CAD build for the part. Positions are in the model's coordinates, mm. A direction names the side the tool comes from. Give positions to 0.01 mm unless a question says otherwise; leave off trailing zeros. Loops run counter-clockwise (first coordinate to the right, second up) from the corner with the lowest first, then second, coordinate; pieces in that order, holes last.
```python
from build123d import *

# Parameters (mm, degrees)
F1_DEPTH = 2
F2_DEPTH = 14
F3_DEPTH = 4
F4_DEPTH = 14
F5_R     = 5


with BuildPart() as f1:
    # F0 (on Front) → F1 (new body)
    with BuildSketch(Plane.XZ):
        Polygon((26.906193, 0), (-25.108696, 0), (-25.108696, -13), (26.906193, -7.798511), align=None)
        Polygon((-25.108696, 10), (-25.108696, 0), (26.906193, 0), (26.906193, 4.798511), align=None)
    extrude(amount=F1_DEPTH)

    # F0 (on Front) → F2 (join)
    with BuildSketch(Plane.XZ):
        Polygon((26.906193, 4.798511), (26.906193, 0), (29.891304, 0), (29.891304, 15), (26.906193, 15), (26.906193, 7.798511), align=None)
    extrude(amount=F2_DEPTH)

    # F0 (on Front) → F3 (join)
    with BuildSketch(Plane.XZ):
        Polygon((-25.108696, 13), (-25.108696, 10), (26.906193, 4.798511), (26.906193, 7.798511), align=None)
    extrude(amount=F3_DEPTH)

    # F0 (on Front) → F4 (join)
    with BuildSketch(Plane.XZ):
        Polygon((29.891304, 0), (26.906193, 0), (26.906193, -7.798511), (26.906193, -15), (29.891304, -15), align=None)
    extrude(amount=F4_DEPTH)

    # F5
    f5_edges = [f1.edges().sort_by_distance(p)[0] for p in [
        (28.398748, -14, -15),
        (28.398748, -14, 15),
    ]]
    fillet(f5_edges, radius=F5_R)


solid = f1.part
```
1. Saw through at D-D, the plane y = -7.25. List the corners of the cut face in (x, z).
Responses:
outline: (26.91, -15) - (29.89, -15) - (29.89, 15) - (26.91, 15) - close
2. Saw through at C-C, the plane x = 18.5. List the corners of the cut face in (y, z), and give its area (3 significant figures).
Responses:
outline: (-4, 5.64) - (-2, 5.64) - (-2, -8.64) - (0, -8.64) - (0, 8.64) - (-4, 8.64) - close
area: 40.6 mm2
3. Drop flat-ended pins along their axis: pin 1 (10 mm diameter, centred on x = -6.5, z = -7, fed in from -Y); pin 2 (1 mm diameter, centred on y = -3, z = -12, fed in from -X); pin 3 (6.5 mm diameter, centred on x = -4.5, z = 8.5, fed in from -Y). Give the stop position or say it passes through.
Responses:
pin 1: stops at y = -2
pin 2: stops at x = 26.91
pin 3: stops at y = -4
4. Probe line 1 along Y through (x, z) = (8.5, 7.75); line 2 along Y through (x, z) = (6.5, 0.5); line 3 along X through (y, z) = (-6.25, 4.25). List the from-to ranges inside material, lowest first.
Responses:
line 1: y = -4 to 0
line 2: y = -2 to 0
line 3: x = 26.91 to 29.89
5. Saw through at B-B, the plane z = 7. List the corners of the cut face in (x, y).
Responses:
outline: (-25.11, -2) - (4.89, -2) - (4.89, -4) - (26.91, -4) - (26.91, -14) - (29.89, -14) - (29.89, 0) - (-25.11, 0) - close
6. Pull direction X, two halves, no side cores. Call faces 1 (the face through (0.535, -0.986, -10.436)), 2 (the face through (0.535, -2.986, 7.436)), 3 (the face through (1, -4, 9)): released by +X, released by -X, zero draft, split by the parting line, or undercut.
Responses:
face 1: undercut
face 2: released by -X
face 3: zero draft
7. Tool access for faces 4 (the face through (1.263, -1.972, 10.363)), 5 (the face through (-5, -2, -1)), 6 (the face through (28, -14, 0)): list every direction of +Z, -Z, +X, -X, +Y, -Y with a clear straight run to the whole face (end or side of a thin tool).
Responses:
face 4: +Z, +Y, -Y
face 5: -Z, -X, -Y
face 6: +Z, -Z, +X, -X, -Y
8. Saw through at A-A, the plane y = -2.75. List the corners of the cut face in (x, z), and give its area (3 significant figures).
Responses:
outline: (-25.11, 10) - (26.91, 4.8) - (26.91, -15) - (29.89, -15) - (29.89, 15) - (26.91, 15) - (26.91, 7.8) - (-25.11, 13) - close
area: 246 mm2
